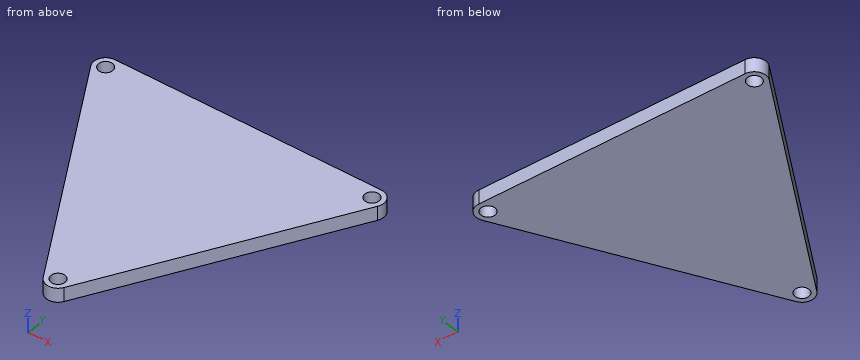
Solid Edge part; units mm, degrees
sketch "Sketch1" plane through (0, 0, 0) normal (0, 0, 1) x (1, 0, 0)
  circle A0 centre (0, -32.8) radius 1.5
  circle A1 centre (-28.0384, 16.188) radius 1.5
  circle A2 centre (28.0384, 16.188) radius 1.5
  line L0 (-30.2081, 14.9461) -> (-2.1697, -34.0419)
  line L1 (2.1697, -34.0419) -> (30.2081, 14.9461)
  line L2 (28.0384, 18.688) -> (-28.0384, 18.688)
  arc A3 (-28.0384, 18.688) -> (-30.2081, 14.9461) centre (-28.0384, 16.188) ccw
  arc A4 (-2.1697, -34.0419) -> (2.1697, -34.0419) centre (0, -32.8) ccw
  arc A5 (30.2081, 14.9461) -> (28.0384, 18.688) centre (28.0384, 16.188) ccw
extrude "Protrusion1" add sketch "Sketch1" along normal blind 3
For this review, take the finished solid that the model builds, in its own axes (mm). Coordinates: 2 decimals unless noted, no trailing zeros. Order: outer loops, then holes, each group sorted by start corner. A loop starts at its lowest first (then second) coordinate and runs counter-clockwise, first axis right, second up. Notation, with made-up numbers: (-30.75, 68) - (13.25, 68) arc R30 ccw to (13.25, 98) - close; hole circle Ø1 at (-35, 25.5). An arc over 180 degrees is marked (long way). Answer as a JSON object with one key per item and string values. Group by question number.
1. We need section A-A on x = 0. State the section outline as (y, z) points.
2. We need section C-C on z = 1.25. State the section outline as (x, y) points, then the cut area to 3 significant figures.
3. We need section B-B on y = -32.8. State the section outline as (x, z) points, then the cut area to 3 significant figures.
4. For probe 1 along Y at (x, z) = (0, 1.6); probe 2 along X at (y, z) = (-31.5, 0.4); probe 3 along Y at (x, z) = (16.5, 0.5), list the stretches that pass through material, from the lowest coordinate up.
5. We need section D-D on y = 14. State the section outline as (x, z) points, then the cut area to 3 significant figures.
6. Clearance check with flat-ended pins moving along their axes: P1, Ø4, axis at x = -28.04, y = 16.19, coming from the -Z side; P2, Ø1.5, axis at y = -23.5, z = 0.5, coming from the -X side. State where each tip first meets the part, or that it passes through.
Final values:
{
 "1": {"outline": "(-35.3, 0) - (-34.3, 0) - (-34.3, 3) - (-35.3, 3) - close; (-31.3, 0) - (18.69, 0) - (18.69, 3) - (-31.3, 3) - close"},
 "2": {"outline": "(-30.21, 14.95) - (-2.17, -34.04) arc R2.5 ccw to (2.17, -34.04) - (30.21, 14.95) arc R2.5 ccw to (28.04, 18.69) - (-28.04, 18.69) arc R2.5 ccw to start; hole circle Ø3 at (-28.04, 16.19); hole circle Ø3 at (0, -32.8); hole circle Ø3 at (28.04, 16.19)", "area": "1,790 mm²"},
 "3": {"outline": "(-2.88, 0) - (-1.5, 0) - (-1.5, 3) - (-2.88, 3) - close; (1.5, 0) - (2.88, 0) - (2.88, 3) - (1.5, 3) - close", "area": "8.28 mm²"},
 "4": {"probe 1": "-35.3 to -34.3, -31.3 to 18.69", "probe 2": "-3.62 to -0.75, 0.75 to 3.62", "probe 3": "-9 to 18.69"},
 "5": {"outline": "(-29.67, 0) - (29.67, 0) - (29.67, 3) - (-29.67, 3) - close", "area": "178 mm²"},
 "6": {"P1": "z = 0", "P2": "x = -8.63"}
}
